```python
from build123d import *

# Parameters (mm, degrees)
BODY_SKETCH_W    = 97
BODY_SKETCH_H    = 95
BODY_DEPTH       = 3
HOLES_DEPTH      = 136.805007271
HOLES_DEPTH_BACK = 136.805007271
HOLES_SKETCH_R   = 1.7
HOLES_SKETCH_R_2 = 25


with BuildPart() as part:
    # Body sketch → Body (new body)
    with BuildSketch(Plane.XY):
        with Locations((48.5, 47.5)):
            Rectangle(BODY_SKETCH_W, BODY_SKETCH_H)
    extrude(amount=BODY_DEPTH)

    # Holes sketch → Holes (cut, two sides: drawn at the far end of the back side and taken through both)
    with BuildSketch(Plane.XY.offset(-HOLES_DEPTH_BACK)):
        with Locations((5.635, 7.495)):
            Circle(HOLES_SKETCH_R)
        with Locations((91.365, 7.495)):
            Circle(HOLES_SKETCH_R)
        with Locations((5.635, 87.505)):
            Circle(HOLES_SKETCH_R)
        with Locations((91.365, 87.505)):
            Circle(HOLES_SKETCH_R)
        with Locations((48.5, 47.5)):
            Circle(HOLES_SKETCH_R_2)
    extrude(amount=HOLES_DEPTH + HOLES_DEPTH_BACK, mode=Mode.SUBTRACT)


solid = part.part
```
Input: part model. Units: mm. Frame: model coordinates. Round coordinates to 2 decimals unless told otherwise and drop trailing zeros. Write each loop counter-clockwise with the first axis right and the second up, starting at its lowest first coordinate (ties: lowest second). Pieces come first, ordered by that corner, then holes. Notation, with made-up numbers: (-10, 25.25) -> (27, 25.25) arc R19 cw to (27, 61.25) -> close; hole circle Ø4 at (2, 31.25). An arc over 180 degrees is marked (long way). Answer as CSV lines item,"result".
1. Mould query, pull axis Y, two halves, no side actions, for faces 1 (the flat face through (0, 47, 1)), 2 (the cylindrical face through (92.935, 6.844, 1.479)), 3 (the flat face through (48, 95, 1)). Classes: +Y half, -Y half, draft (parallel to the pull), parting line (faces both ways), or undercut.
Geometry says:
face 1,"draft"
face 2,"undercut"
face 3,"+Y half"
2. Section B-B (y = 52). Return the cut outline in (x, z), plus the area to 3 significant figures.
Geometry says:
outline,"(0, 0) -> (23.91, 0) -> (23.91, 3) -> (0, 3) -> close; (73.09, 0) -> (97, 0) -> (97, 3) -> (73.09, 3) -> close"
area,"143 mm^2"
3. Section A-A (x = 48.5). Return the cut outline in (y, z), plus the area to 3 significant figures.
Geometry says:
outline,"(0, 0) -> (22.5, 0) -> (22.5, 3) -> (0, 3) -> close; (72.5, 0) -> (95, 0) -> (95, 3) -> (72.5, 3) -> close"
area,"135 mm^2"
4. Contact query for a flat-ended pin moving along its axis: P1, Ø2, axis at x = 91.365, y = 87.505, coming from the +Z side. Output: stop coordinate, or through.
Geometry says:
P1,"passes through"
5. Ray query, L1, parallel to X at y = 47.5, z = 1.15; L2, parallel to Y at x = 48.5, z = 1.55; L3, parallel to X at y = 51.5, z = 1.35. Return the intervals inside material, ascending. Write a range as [from, to].
Geometry says:
L1,"x = [0, 23.5], [73.5, 97]"
L2,"y = [0, 22.5], [72.5, 95]"
L3,"x = [0, 23.82], [73.18, 97]"
6. Section C-C (z = 0.55). Return the cut outline in (x, y) (3 decimals).
Geometry says:
outline,"(0, 0) -> (97, 0) -> (97, 95) -> (0, 95) -> close; hole circle Ø3.4 at (5.635, 7.495); hole circle Ø3.4 at (5.635, 87.505); hole circle Ø50 at (48.5, 47.5); hole circle Ø3.4 at (91.365, 7.495); hole circle Ø3.4 at (91.365, 87.505)"
